```python
from build123d import *

# Parameters (mm, degrees)
SKETCH1_W           = 23.339745962
SKETCH1_H           = 77.847771952
EXTRUDE1_DEPTH      = 2
SKETCH2_W           = 23.339745962
SKETCH2_H           = 58.47295833
EXTRUDE2_DEPTH      = 2
EXTRUDE3_DEPTH      = 2
EXTRUDE4_DEPTH      = 2
SKETCH5_W           = 29.172294857
SKETCH5_H           = 114.252589879
CUT_EXTRUDE1_DEPTH  = 2
SKETCH6_W           = 35.17541313
SKETCH6_H           = 36.355570025
CUT_EXTRUDE3_DEPTH  = 9
SKETCH7_W           = 29.640366785
SKETCH7_H           = 86.495658127
CUT_EXTRUDE4_DEPTH  = 9
SKETCH8_W           = 29.536232552
SKETCH8_H           = 67.327773858
CUT_EXTRUDE5_DEPTH  = 9
SKETCH9_W           = 23.303500438
SKETCH9_H           = 17.745035166
CUT_EXTRUDE6_DEPTH  = 9
SKETCH10_W          = 29.605950058
SKETCH10_H          = 24.209977647
CUT_EXTRUDE7_DEPTH  = 9
SKETCH11_W          = 17.28028661
SKETCH11_H          = 57.043927735
CUT_EXTRUDE8_DEPTH  = 9
SKETCH12_W          = 46.644962208
SKETCH12_H          = 26.527348651
CUT_EXTRUDE9_DEPTH  = 9
SKETCH13_W          = 27.90261226
SKETCH13_H          = 36.830907155
CUT_EXTRUDE10_DEPTH = 9
CUT_EXTRUDE11_DEPTH = 9
CUT_EXTRUDE12_DEPTH = 9
EXTRUDE5_REACH      = 108.706
SKETCH16_R          = 1.6
SKETCH18_R          = 3
CUT_EXTRUDE13_DEPTH = 16
CUT_EXTRUDE14_DEPTH = 46


with BuildPart() as part:
    # Sketch1 → Extrude1 (new body)
    with BuildSketch(Plane.XY):
        with Locations((11.669872981, -62.635077412)):
            Rectangle(SKETCH1_W, SKETCH1_H)
    extrude(amount=EXTRUDE1_DEPTH)

    # Sketch2 → Extrude2 (add)
    with BuildSketch(Plane(origin=(0, -0.312184271, -2.780754984), x_dir=(1, 0, 0), z_dir=(-1.8145207558717603e-15, 0.11156514837203096, 0.9937571220719512))):
        with Locations((11.669872981, 3.838577658)):
            Rectangle(SKETCH2_W, SKETCH2_H)
    extrude(amount=EXTRUDE2_DEPTH)

    # Sketch3 → Extrude3 (add)
    with BuildSketch(Plane(origin=(17.504809472, 0, 10.106406461), x_dir=(0.49999999999999906, -1.634548474587185e-15, -0.8660254037844393), z_dir=(0.8660254037844392, -2.831121005419217e-15, 0.499999999999999))):
        Polygon((7.883442522, -104.490571733), (28.990381057, -88.148722114), (28.990381057, -25.920882689), (7.883442522, -23.352575413), align=None)
    extrude(amount=EXTRUDE3_DEPTH)

    # Sketch4 → Extrude4 (add)
    with BuildSketch(Plane(origin=(16.293142957, 1.049476669, 9.348124653), x_dir=(0.49585100083824124, 0.031938838189501655, -0.8678200824956861), z_dir=(0.8660254037844394, 0.055782574186015135, 0.49687856103597455))):
        Polygon((16.15670827, 37.302716602), (33.476734925, 13.886588158), (28.056650386, -27.924204291), (7.502507009, -29.456207578), align=None)
    extrude(amount=EXTRUDE4_DEPTH)

    # Sketch5 → Cut-Extrude1 (cut)
    with BuildSketch(Plane(origin=(32, 0, 0), x_dir=(0, 0, -1), z_dir=(1, 0, 0))):
        with Locations((10.907999104, -37.350448714)):
            Rectangle(SKETCH5_W, SKETCH5_H)
    extrude(amount=CUT_EXTRUDE1_DEPTH, mode=Mode.SUBTRACT)

    # Sketch6 → Cut-Extrude3 (cut)
    with BuildSketch(Plane(origin=(0, -100.294881076, 11.25970626), x_dir=(1, 0, 0), z_dir=(0, -0.9937571220719427, 0.11156514837210559))):
        with Locations((14.876045987, -2.775102741)):
            Rectangle(SKETCH6_W, SKETCH6_H)
    extrude(amount=CUT_EXTRUDE3_DEPTH, mode=Mode.SUBTRACT)

    # Sketch7 → Cut-Extrude4 (cut)
    with BuildSketch(Plane.XY.offset(2)):
        with Locations((12.797447922, -61.090112125)):
            Rectangle(SKETCH7_W, SKETCH7_H)
    extrude(amount=CUT_EXTRUDE4_DEPTH, mode=Mode.SUBTRACT)

    # Sketch8 → Cut-Extrude5 (cut)
    with BuildSketch(Plane(origin=(0, -0.089053974, -0.79324074), x_dir=(1, 0, 0), z_dir=(-1.815565503199705e-15, 0.11156514837203098, 0.9937571220719512))):
        with Locations((12.836169201, 6.237775634)):
            Rectangle(SKETCH8_W, SKETCH8_H)
    extrude(amount=CUT_EXTRUDE5_DEPTH, mode=Mode.SUBTRACT)

    # Sketch9 → Cut-Extrude6 (cut)
    with BuildSketch(Plane(origin=(19.236860279, 0, 11.106406461), x_dir=(0.499999999999999, -1.6472663592524059e-15, -0.8660254037844393), z_dir=(0.8660254037844393, -2.8531490278241828e-15, 0.499999999999999))):
        with Locations((15.539372555, -25.628375436)):
            Rectangle(SKETCH9_W, SKETCH9_H)
    extrude(amount=CUT_EXTRUDE6_DEPTH, mode=Mode.SUBTRACT)

    # Sketch10 → Cut-Extrude7 (cut)
    with BuildSketch(Plane(origin=(18.025193764, 1.161041817, 10.341881775), x_dir=(0.49585100083824124, 0.03193883818950166, -0.8678200824956862), z_dir=(0.8660254037844393, 0.05578257418601514, 0.49687856103597444))):
        with Locations((15.868735202, -22.435122808)):
            Rectangle(SKETCH10_W, SKETCH10_H)
    extrude(amount=CUT_EXTRUDE7_DEPTH, mode=Mode.SUBTRACT)

    # Sketch11 → Cut-Extrude8 (cut)
    with BuildSketch(Plane(origin=(0, 32.868573281, -3.690023622), x_dir=(1, 0, 0), z_dir=(0, 0.9937571220719428, -0.11156514837210517))):
        with Locations((25.498335125, 2.54094703)):
            Rectangle(SKETCH11_W, SKETCH11_H)
    extrude(amount=CUT_EXTRUDE8_DEPTH, mode=Mode.SUBTRACT)

    # Sketch12 → Cut-Extrude9 (cut)
    with BuildSketch(Plane(origin=(31.826729192, 18.260456719, -2.050028642), x_dir=(-0.048384463847340485, -0.027760389785225534, -0.9984429399906526), z_dir=(0.8660254037844403, 0.496878561035969, -0.055782574186050725))):
        with Locations((12.073297204, 7.763321363)):
            Rectangle(SKETCH12_W, SKETCH12_H)
    extrude(amount=CUT_EXTRUDE9_DEPTH, mode=Mode.SUBTRACT)

    # Sketch13 → Cut-Extrude10 (cut)
    with BuildSketch(Plane(origin=(61.206591805, -35.117033668, 3.942449301), x_dir=(0.048384463847343365, -0.027760389785227164, -0.9984429399906524), z_dir=(0.8660254037844402, -0.49687856103596856, 0.055782574186054035))):
        with Locations((11.882531158, -68.145692396)):
            Rectangle(SKETCH13_W, SKETCH13_H)
    extrude(amount=CUT_EXTRUDE10_DEPTH, mode=Mode.SUBTRACT)

    # Sketch14 → Cut-Extrude11 (cut)
    with BuildSketch(Plane.XY.offset(2)):
        with BuildLine():
            Line((-5.730960927, -24.969609587), (9, -24.969609587))
            ThreePointArc((9, -24.969609587), (15, -30.969609587), (9, -36.969609587))
            Line((9, -36.969609587), (-5.730960927, -36.969609587))
            ThreePointArc((-5.730960927, -36.969609587), (-11.730960927, -30.969609587), (-5.730960927, -24.969609587))
        make_face()
    extrude(amount=-CUT_EXTRUDE11_DEPTH, mode=Mode.SUBTRACT)

    # Sketch15 → Cut-Extrude12 (cut)
    with BuildSketch(Plane(origin=(18.025193764, 1.161041817, 10.341881775), x_dir=(0.49585100083824163, 0.03193883818950172, -0.8678200824956859), z_dir=(0.866025403784439, 0.055782574186015205, 0.49687856103597494))):
        with BuildLine():
            Line((20.949277707, 6.423782658), (31.529743864, 5.052198489))
            ThreePointArc((31.529743864, 5.052198489), (36.708608329, -1.669361066), (29.987048774, -6.848225531))
            Line((29.987048774, -6.848225531), (19.406582616, -5.476641362))
            ThreePointArc((19.406582616, -5.476641362), (14.227718152, 1.244918193), (20.949277707, 6.423782658))
        make_face()
    extrude(amount=-CUT_EXTRUDE12_DEPTH, mode=Mode.SUBTRACT)

    # Sketch16 → Extrude5 (add, up to next)
    with BuildSketch(Plane(origin=(0, -2.320356941, -20.668383181), x_dir=(1, 0, 0), z_dir=(-1.8077100882975075e-15, 0.111565148372031, 0.9937571220719512)), mode=Mode.PRIVATE) as extrude5_sk1:
        with BuildLine():
            Line((29.8, 17.4855686), (29.8, 11.55156303))
            ThreePointArc((29.8, 11.55156303), (21.025378802, 14.298044274), (29.072366829, 18.745866221))
            Line((29.072366829, 18.745866221), (29.8, 17.4855686))
        make_face()
        with Locations((26, 14.801178392)):
            Circle(SKETCH16_R, mode=Mode.SUBTRACT)
    extrude5_tool1 = extrude(extrude5_sk1.sketch, amount=EXTRUDE5_REACH, mode=Mode.PRIVATE) - part.part
    # Sketch16 → Extrude5 (add, up to next)
    with BuildSketch(Plane(origin=(0, -2.320356941, -20.668383181), x_dir=(1, 0, 0), z_dir=(-1.8077100882975075e-15, 0.111565148372031, 0.9937571220719512)), mode=Mode.PRIVATE) as extrude5_sk2:
        with BuildLine():
            Line((2.2, -72.299459365), (2.2, -78.798690089))
            ThreePointArc((2.2, -78.798690089), (11, -75.549074727), (2.2, -72.299459365))
        make_face()
        with Locations(Location((6, -75.549074727, 0), (0, 0, 270))):
            Circle(SKETCH16_R, mode=Mode.SUBTRACT)
    extrude5_tool2 = extrude(extrude5_sk2.sketch, amount=EXTRUDE5_REACH, mode=Mode.PRIVATE) - part.part
    # Sketch16 → Extrude5 (add, up to next)
    with BuildSketch(Plane(origin=(0, -2.320356941, -20.668383181), x_dir=(1, 0, 0), z_dir=(-1.8077100882975075e-15, 0.111565148372031, 0.9937571220719512)), mode=Mode.PRIVATE) as extrude5_sk3:
        with BuildLine():
            Line((29.8, -43.867117974), (29.8, -50.366348697))
            ThreePointArc((29.8, -50.366348697), (21, -47.116733335), (29.8, -43.867117974))
        make_face()
        with Locations(Location((26, -47.116733335, 0), (0, 0, 356.314545866))):
            Circle(SKETCH16_R, mode=Mode.SUBTRACT)
    extrude5_tool3 = extrude(extrude5_sk3.sketch, amount=EXTRUDE5_REACH, mode=Mode.PRIVATE) - part.part
    add(extrude5_tool1.solids().sort_by_distance((29.320823, 15.616079, -22.682035))[0])
    add(extrude5_tool2.solids().sort_by_distance((10.866793, -77.397788, -12.239739))[0])
    add(extrude5_tool3.solids().sort_by_distance((29.666793, -49.142946, -15.411798))[0])

    # Sketch18 → Cut-Extrude13 (cut)
    with BuildSketch(Plane(origin=(0, -0.089053974, -0.79324074), x_dir=(1, 0, 0), z_dir=(-1.8077100882975075e-15, 0.111565148372031, 0.9937571220719512))):
        with Locations(Location((26, 14.801178392, 0), (0, 0, 270))):
            Circle(SKETCH18_R)
        with Locations(Location((26, -47.116733335, 0), (0, 0, 270))):
            Circle(SKETCH18_R)
        with Locations(Location((6, -75.549074727, 0), (0, 0, 270))):
            Circle(SKETCH18_R)
    extrude(amount=-CUT_EXTRUDE13_DEPTH, mode=Mode.SUBTRACT)

    # Sketch19 → Cut-Extrude14 (cut)
    with BuildSketch(Plane.XY.offset(2)):
        with BuildLine():
            Line((-9.54644603, -56.58750618), (4, -56.58750618))
            ThreePointArc((4, -56.58750618), (8, -60.58750618), (4, -64.58750618))
            Line((4, -64.58750618), (-9.54644603, -64.58750618))
            ThreePointArc((-9.54644603, -64.58750618), (-13.54644603, -60.58750618), (-9.54644603, -56.58750618))
        make_face()
    extrude(amount=-CUT_EXTRUDE14_DEPTH, mode=Mode.SUBTRACT)


solid = part.part
```
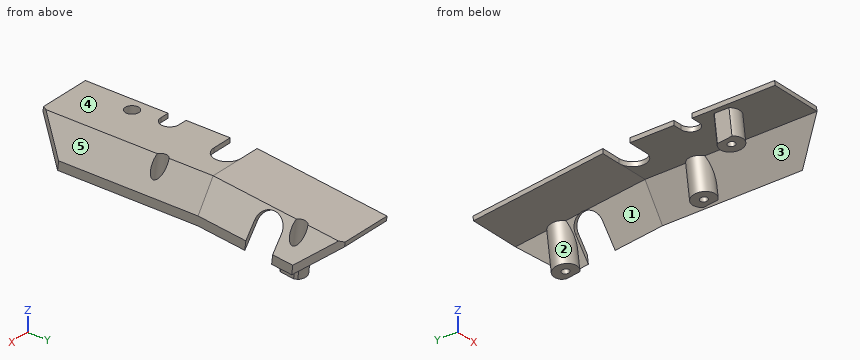
Here's how the part is built. I have some questions about the finished solid (model axes, mm). Face numbers are marked on the shaded views. A direction names the side the tool comes from. Round coordinates to 2 decimals unless told otherwise and drop trailing zeros. Loops run counter-clockwise (first coordinate to the right, second up) from the corner with the lowest first, then second, coordinate; pieces in that order, holes last.
1. Suppose I cut it at A-A, the plane x = 16.5. Please give me the cut outline in (y, z), and give its area (3 significant figures).
Answers:
outline: (-101.56, 0) - (-25.08, 0) - (32.56, -6.47) - (32.78, -4.48) - (-24.97, 2) - (-101.33, 2) - close
area: 269 mm2
2. For the marked faces 1 and 2, which set-ups out of +Z, -Z, +X, -X, +Y, -Y let a thin tool reach every point of the face, with its end or its side?
Answers:
face 1: -Z, -X
face 2: none
3. Will these pins go through, and if not, where does the flat tip stop? pin 1 (1.5 mm diameter, centred on y = -81.5, z = -9.5, fed in from -X); pin 2 (6 mm diameter, centred on x = 23.5, y = -3, fed in from -Z); pin 3 (1 mm diameter, centred on x = 1, z = 1, fed in from -Y).
Answers:
pin 1: stops at x = 2.56
pin 2: stops at z = -7.7
pin 3: stops at y = -101.5
4. If I drill on probe 1 along Y at (x, z) = (26.5, -12); probe 2 along X at (y, z) = (11.5, -20.25); probe 3 along Y at (x, z) = (6, -10.5), over which ranges is the centre line in solid material (lowest first)?
Answers:
probe 1: y = -53.77 to -50.29, -47.23 to -43.75, 8.54 to 10.57, 16.52 to 18.55
probe 2: x = 21.13 to 24.85, 27.15 to 29.8
probe 3: y = -82.23 to -78.81, -75.59 to -72.17
5. Thinking about a two-plate mould opening in X: for the marked faces 3, 4 and 5, which applies, released by +X, released by -X, zero draft, split by the parting line, or undercut?
Answers:
face 3: undercut
face 4: zero draft
face 5: released by +X
6. Suppose I cut it at B-B, the plane y = 21.5. Please give me the cut outline in (x, z), and give its area (3 significant figures).
Answers:
outline: (0, -5.23) - (23.34, -5.23) - (29.11, -15.3) - (29.35, -11.68) - (24.49, -3.22) - (0, -3.22) - close
area: 69.5 mm2
